Here's how the part is built. I have some questions about the finished solid (model axes, mm). Face numbers are marked on the shaded views. A direction names the side the tool comes from. Give positions to 0.01 mm unless a question says otherwise; leave off trailing zeros. Write each loop counter-clockwise with the first axis right and the second up, starting at its lowest first coordinate (ties: lowest second). Pieces come first, ordered by that corner, then holes. Notation, with made-up numbers: M 22,84 L 44,84 A25 cw 44,118 Z; hole C 76.25,5 d11. An arc over 180 degrees is marked long. Answer as CSV lines item,"result". Start each with the question number.
Q1. Suppose I cut it at B-B (y = 11.5). Write out the boundary of the cut face in (x, z), then the cut area to 3 significant figures.
Q2. For pin 1 (3 mm diameter, centred on x = -38.5, z = -6.5, fed in from +Y); pin 2 (2 mm diameter, centred on y = 12.5, z = 1.5, fed in from +X); pin 3 (5 mm diameter, centred on x = 35, z = -7, fed in from +Y); pin 4 (0.8 mm diameter, centred on y = 17.5, z = -6, fed in from -X), each with a flat end and sliding along its axis, tell me the tip position at first contact or that it passes through.
Q3. On a 3-axis mill with a long thin cutter (end or side, diameter ignored), from which of +Z, -Z, +X, -X, +Y, -Y can I reach the whole of each face in a straight line? I mean the marked faces 1, 2 and 3. Say none if no direction works.
Q4. Suppose I cut it at C-C (x = -14.5). Write out the boundary of the cut face in (y, z), then the cut area to 3 significant figures.
Q5. Suppose I cut it at A-A (z = 1). Write out the boundary of the cut face in (x, y), then the cut area to 3 significant figures.
Q6. If I drill on line 1 along X through (y, z) = (6, 18); line 2 along X through (y, z) = (15.25, -12); line 3 along Z through (x, y) = (-50.5, 13), over which ranges is the centre line in solid material (lowest first)?
Q7. Thinking about a two-plate mould opening in Z: for the marked faces 4, 5 and 6, which applies, +Z half, -Z half, draft (parallel to the pull), parting line (faces both ways), or undercut?
Q8. Suppose I cut it at D-D (x = 46). Write out the boundary of the cut face in (y, z), then the cut area to 3 significant figures.
```python
from build123d import *

# Parameters (mm, degrees)
BOSS_EXTRUDE1_DEPTH = 18
SKETCH2_R           = 8.516680521
BOSS_EXTRUDE2_DEPTH = 17.99267
SKETCH3_W           = 78.234373806
SKETCH3_H           = 54.777100321
CUT_EXTRUDE1_DEPTH  = 1
SKETCH4_W           = 15.862685655
SKETCH4_H           = 14.014084995
SKETCH4_W_2         = 19.585195724
BOSS_EXTRUDE3_DEPTH = 1
SKETCH5_W           = 4.110560002
SKETCH5_H           = 9.404487674
CUT_EXTRUDE2_DEPTH  = 9.590155657


with BuildPart() as part:
    # Sketch1 → Boss-Extrude1 (new body)
    with BuildSketch(Plane(origin=(0, 0, 0), x_dir=(1, 0, 0), z_dir=(0, 1, 0))):
        Polygon((-55.602513221, 28.358711105), (-55.602513221, 19.768555449), (-47.518849821, 19.768555449), (-47.518849821, -10.055277405), (-55.602513221, -10.055277405), (-55.602513221, -36.571359429), (60.697934404, -36.571359429), (60.697934404, -28.748459365), (42.705264255, -28.748459365), (42.705264255, 13.755964318), (42.705264255, 28.358711105), align=None)
    extrude(amount=BOSS_EXTRUDE1_DEPTH)

    # Sketch2 → Boss-Extrude2 (add)
    with BuildSketch(Plane(origin=(42.705264255, 0, 0), x_dir=(0, 0, -1), z_dir=(1, 0, 0))):
        with Locations(Location((18.133704787, 8.780998405, 0), (0, 0, 180))):  # turned: the seam where the file's is
            Circle(SKETCH2_R)
    extrude(amount=BOSS_EXTRUDE2_DEPTH)

    # Sketch3 → Cut-Extrude1 (cut)
    with BuildSketch(Plane(origin=(0, 18, 0), x_dir=(1, 0, 0), z_dir=(0, 1, 0))):
        with Locations((-2.172142095, -4.144542808)):
            Rectangle(SKETCH3_W, SKETCH3_H)
    extrude(amount=-CUT_EXTRUDE1_DEPTH, mode=Mode.SUBTRACT)

    # Sketch4 → Boss-Extrude3 (add)
    with BuildSketch(Plane(origin=(0, 17, 0), x_dir=(1, 0, 0), z_dir=(0, 1, 0))):
        with Locations((25.510271921, -22.585660372)):
            Rectangle(SKETCH4_W, SKETCH4_H)
        with Locations((-29.019306935, -22.585660372)):
            Rectangle(SKETCH4_W_2, SKETCH4_H)
    extrude(amount=BOSS_EXTRUDE3_DEPTH)

    # Sketch5 → Cut-Extrude2 (cut, through all)
    with BuildSketch(Plane.XY.offset(-19.768555449)):
        with Locations((-49.574129822, 8.723143931)):
            Rectangle(SKETCH5_W, SKETCH5_H)
    extrude(amount=-CUT_EXTRUDE2_DEPTH, mode=Mode.SUBTRACT)


solid = part.part
```
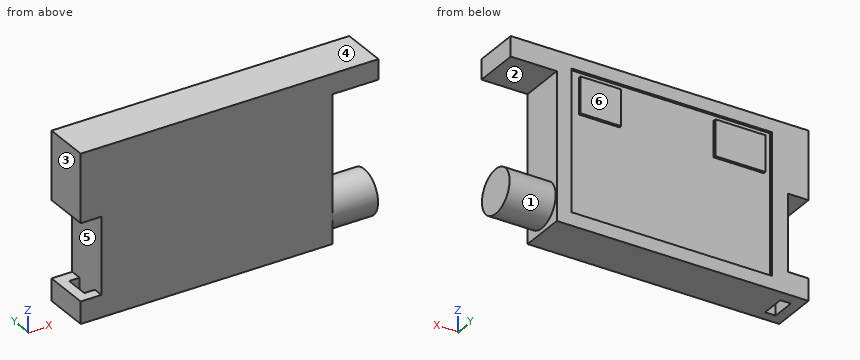
Resolved:
1,outline,"M -55.6,-28.36 L -51.63,-28.36 L -51.63,-19.77 L -55.6,-19.77 Z; M -55.6,10.06 L -47.52,10.06 L -47.52,-28.36 L 42.71,-28.36 L 42.71,-26.2 L 60.7,-26.2 L 60.7,-10.06 L 42.71,-10.06 L 42.71,28.75 L 60.7,28.75 L 60.7,36.57 L -55.6,36.57 Z"
1,area,"6,540 mm^2"
2,pin 1,"y = 17"
2,pin 2,"x = 42.71"
2,pin 3,"y = 18"
2,pin 4,"x = -47.52"
3,face 1,"+X"
3,face 2,"+X, +Y, -Y"
3,face 3,"+Z, -Z, -X, +Y, -Y"
4,outline,"M 0,-28.36 L 18,-28.36 L 18,-23.24 L 17,-23.24 L 17,31.53 L 18,31.53 L 18,36.57 L 0,36.57 Z"
4,area,"1,110 mm^2"
5,outline,"M -47.52,0 L 42.71,0 L 42.71,18 L 36.95,18 L 36.95,17 L -41.29,17 L -41.29,18 L -47.52,18 Z"
5,area,"1,550 mm^2"
6,line 1,"-55.6 to 42.71"
6,line 2,"-47.52 to 42.71"
6,line 3,"10.06 to 36.57"
7,face 4,"+Z half"
7,face 5,"undercut"
7,face 6,"draft"
8,outline,"M 0,28.75 L 18,28.75 L 18,36.57 L 0,36.57 Z; C 8.78,-18.13 d17.03"
8,area,"369 mm^2"
